from build123d import *

# Parameters (mm, degrees)
CROQUIS1_W              = 250
CROQUIS1_H              = 350
SALIENTE_EXTRUIR2_DEPTH = 15
CROQUIS2_W              = 30
CROQUIS2_H              = 30
SALIENTE_EXTRUIR3_DEPTH = 300
CROQUIS3_W              = 250
CROQUIS3_H              = 350
SALIENTE_EXTRUIR4_DEPTH = 5
CROQUIS7_W              = 70
CROQUIS7_H              = 5
CORTAR_EXTRUIR1_DEPTH   = 20
CROQUIS8_W              = 250
CROQUIS8_H              = 320
SALIENTE_EXTRUIR5_DEPTH = 5
CROQUIS9_W              = 250
CROQUIS9_H              = 320
SALIENTE_EXTRUIR6_DEPTH = 5


with BuildPart() as part:
    # Croquis1 → Saliente-Extruir2 (new body)
    with BuildSketch(Plane.XY):
        Rectangle(CROQUIS1_W, CROQUIS1_H)
    extrude(amount=SALIENTE_EXTRUIR2_DEPTH)

    # Croquis2 → Saliente-Extruir3 (add)
    with BuildSketch(Plane.XY.offset(15)):
        with Locations((-110, 160)):
            Rectangle(CROQUIS2_W, CROQUIS2_H)
        with Locations((110, 160)):
            Rectangle(CROQUIS2_W, CROQUIS2_H)
        with Locations((-110, -160)):
            Rectangle(CROQUIS2_W, CROQUIS2_H)
        with Locations((110, -160)):
            Rectangle(CROQUIS2_W, CROQUIS2_H)
    extrude(amount=SALIENTE_EXTRUIR3_DEPTH)

    # Croquis3 → Saliente-Extruir4 (add)
    with BuildSketch(Plane.XY.offset(315)):
        Rectangle(CROQUIS3_W, CROQUIS3_H)
    extrude(amount=SALIENTE_EXTRUIR4_DEPTH)

    # Croquis7 → Cortar-Extruir1 (cut)
    with BuildSketch(Plane(origin=(0, 0, 0), x_dir=(-1, 0, 0), z_dir=(0, 0, -1))):
        with Locations((60, 132.5)):
            Rectangle(CROQUIS7_W, CROQUIS7_H)
        with Locations((-60, 132.5)):
            Rectangle(CROQUIS7_W, CROQUIS7_H)
        with Locations((60, 112.5)):
            Rectangle(CROQUIS7_W, CROQUIS7_H)
        with Locations((60, 92.5)):
            Rectangle(CROQUIS7_W, CROQUIS7_H)
        with Locations((60, 72.5)):
            Rectangle(CROQUIS7_W, CROQUIS7_H)
        with Locations((60, 52.5)):
            Rectangle(CROQUIS7_W, CROQUIS7_H)
        with Locations((60, 32.5)):
            Rectangle(CROQUIS7_W, CROQUIS7_H)
        with Locations((60, 12.5)):
            Rectangle(CROQUIS7_W, CROQUIS7_H)
        with Locations((60, -7.5)):
            Rectangle(CROQUIS7_W, CROQUIS7_H)
        with Locations((60, -27.5)):
            Rectangle(CROQUIS7_W, CROQUIS7_H)
        with Locations((60, -47.5)):
            Rectangle(CROQUIS7_W, CROQUIS7_H)
        with Locations((-60, 112.5)):
            Rectangle(CROQUIS7_W, CROQUIS7_H)
        with Locations((-60, 92.5)):
            Rectangle(CROQUIS7_W, CROQUIS7_H)
        with Locations((-60, 72.5)):
            Rectangle(CROQUIS7_W, CROQUIS7_H)
        with Locations((-60, 52.5)):
            Rectangle(CROQUIS7_W, CROQUIS7_H)
        with Locations((-60, 32.5)):
            Rectangle(CROQUIS7_W, CROQUIS7_H)
        with Locations((-60, 12.5)):
            Rectangle(CROQUIS7_W, CROQUIS7_H)
        with Locations((-60, -7.5)):
            Rectangle(CROQUIS7_W, CROQUIS7_H)
        with Locations((-60, -27.5)):
            Rectangle(CROQUIS7_W, CROQUIS7_H)
        with Locations((-60, -47.5)):
            Rectangle(CROQUIS7_W, CROQUIS7_H)
        with Locations((-60, -67.5)):
            Rectangle(CROQUIS7_W, CROQUIS7_H)
        with Locations((60, -67.5)):
            Rectangle(CROQUIS7_W, CROQUIS7_H)
        with Locations((-60, -87.5)):
            Rectangle(CROQUIS7_W, CROQUIS7_H)
        with Locations((60, -87.5)):
            Rectangle(CROQUIS7_W, CROQUIS7_H)
        with Locations((-60, -107.5)):
            Rectangle(CROQUIS7_W, CROQUIS7_H)
        with Locations((60, -107.5)):
            Rectangle(CROQUIS7_W, CROQUIS7_H)
        with Locations((-60, -127.5)):
            Rectangle(CROQUIS7_W, CROQUIS7_H)
        with Locations((60, -127.5)):
            Rectangle(CROQUIS7_W, CROQUIS7_H)
    extrude(amount=-CORTAR_EXTRUIR1_DEPTH, mode=Mode.SUBTRACT)

    # Croquis8 → Saliente-Extruir5 (add)
    with BuildSketch(Plane.XZ.offset(175)):
        with Locations((0, 160)):
            Rectangle(CROQUIS8_W, CROQUIS8_H)
    extrude(amount=-SALIENTE_EXTRUIR5_DEPTH)

    # Croquis9 → Saliente-Extruir6 (add)
    with BuildSketch(Plane(origin=(0, 175, 0), x_dir=(1, 0, 0), z_dir=(0, 1, 0))):
        with Locations((0, -160)):
            Rectangle(CROQUIS9_W, CROQUIS9_H)
    extrude(amount=-SALIENTE_EXTRUIR6_DEPTH)


solid = part.part
Source: CAD feature listing. Evaluate the final solid. Frame: model axes, mm. A direction names the side the tool comes from. Coordinates: 2 decimals unless noted, no trailing zeros. Loops run counter-clockwise (first coordinate to the right, second up) from the corner with the lowest first, then second, coordinate; pieces in that order, holes last. Notation, with made-up numbers: M -13,74.5 L -2,74.5 A23 ccw -2,100.5 Z; hole C 38.5,37.5 d11. An arc over 180 degrees is marked long. Answer in a Markdown table with one row per item.
Q1. Ray query, probe 1 along Z at (x, y) = (31, 27.5); probe 2 along Y at (x, z) = (-81, 111); probe 3 along Y at (x, z) = (111, 58.5). Return the intervals inside material, ascending. Write a range as from..to.
Answers below:
| item | result |
|---|---|
| probe 1 | z = 0..15, 315..320 |
| probe 2 | y = -175..-170, 170..175 |
| probe 3 | y = -175..-145, 145..175 |
Q2. Section B-B on x = 19. Return the cut outline in (y, z), plus the area to 3 significant figures.
Answers below:
| item | result |
|---|---|
| outline | M -175,0 L 175,0 L 175,320 L -175,320 Z; hole M -170,15 L 170,15 L 170,315 L -170,315 Z |
| area | 10,000 mm^2 |
Q3. Section C-C on z = 73. Return the cut outline in (x, y), plus the area to 3 significant figures.
Answers below:
| item | result |
|---|---|
| outline | M -125,-175 L 125,-175 L 125,-145 L 95,-145 L 95,-170 L -95,-170 L -95,-145 L -125,-145 Z; M -125,145 L -95,145 L -95,170 L 95,170 L 95,145 L 125,145 L 125,175 L -125,175 Z |
| area | 5,500 mm^2 |
Q4. Set-up query: faces 1 (the flat face through (-60, 75, 7)), 2 (the flat face through (-2, 175, 158)). Return all of +Z, -Z, +X, -X, +Y, -Y with unobstructed straight access to the full face (end or side cutting, diameter ignored); none if empty.
Answers below:
| item | result |
|---|---|
| face 1 | -Z |
| face 2 | +Z, -Z, +X, -X, +Y |
Q5. Section D-D on y = 153. Return the cut outline in (x, z).
Answers below:
| item | result |
|---|---|
| outline | M -125,0 L 125,0 L 125,320 L -125,320 Z; hole M -95,15 L 95,15 L 95,315 L -95,315 Z |
Q6. Section A-A on y = 104. Return the cut outline in (x, z).
Answers below:
| item | result |
|---|---|
| outline | M -125,0 L 125,0 L 125,15 L -125,15 Z; M -125,315 L 125,315 L 125,320 L -125,320 Z |
Q7. First-contact query: pin 1 (8 mm diameter, centred on x = -11, y = 49, fed in from -Z). Flat tip, straight axial feed; report the tip coordinate or a pass-through.
Answers below:
| item | result |
|---|---|
| pin 1 | stops at z = 0 |
Q8. Draft query along Y for faces 3 (the flat face through (-2, -175, 158)), 4 (the flat face through (125, -1, 5)), 5 (the flat face through (110, 145, 163)). Return one class per face: pulls with the +Y half, pulls with the -Y half, needs draft (parallel to the pull), parting line crosses it, or undercut.
Answers below:
| item | result |
|---|---|
| face 3 | pulls with the -Y half |
| face 4 | needs draft |
| face 5 | undercut |
